Autodesk Fusion 360 part; units mm, degrees
sketch "Sketch1" plane through (0, 0, 0) normal (0, 0, 1) x (1, 0, 0)
  line L0 (12.75, -12.75) -> (-12.75, -12.75)
  line L1 (-12.75, -12.75) -> (-12.75, 12.75)
  line L2 (-12.75, 12.75) -> (12.75, 12.75)
  line L3 (12.75, 12.75) -> (12.75, -12.75)
  line L4 (12.75, -12.75) -> (-12.75, 12.75) construction
  line L5 (-12.75, -12.75) -> (12.75, 12.75) construction
  line L6 (-0.75, 12.75) -> (0.75, 12.75)
  line L7 (0.75, 12.75) -> (0.75, 42.75)
  line L8 (0.75, 42.75) -> (-0.75, 42.75)
  line L9 (-0.75, 42.75) -> (-0.75, 12.75)
  dimension "d1" = 25.5
  dimension "d2" = 25.5
  dimension "d3" = 1.5
  dimension "d4" = 30
  dimension "d5" = 0.75
extrude "Extrude1" add sketch "Sketch1" along normal blind 10 makes body 1
sketch "Sketch2" plane through (0, 0, 10) normal (0, 0, 1) x (-1, 0, 0)
  line L0 (-0.75, -12.75) -> (-0.75, -42.75)
  line L1 (-0.75, -42.75) -> (0.75, -42.75)
  line L2 (0.75, -42.75) -> (0.75, -12.75)
  line L3 (0.75, -12.75) -> (12.75, -12.75)
  line L4 (12.75, -12.75) -> (12.75, 12.75)
  line L5 (12.75, 12.75) -> (-12.75, 12.75)
  line L6 (-12.75, 12.75) -> (-12.75, -12.75)
  line L7 (-12.75, -12.75) -> (-0.75, -12.75)
  line L8 (-15, 15) -> (15, 15)
  line L9 (15, 15) -> (15, -15)
  line L10 (15, -15) -> (-15, -15)
  line L11 (-15, -15) -> (-15, 15)
  line L12 (-15, 15) -> (15, -15) construction
  line L13 (15, 15) -> (-15, -15) construction
  line L14 (-22.5, 15) -> (22.5, 15)
  line L15 (22.5, 15) -> (22.5, -15)
  line L16 (22.5, -15) -> (-22.5, -15)
  line L17 (-22.5, -15) -> (-22.5, 15)
  line L18 (-22.5, 15) -> (22.5, -15) construction
  line L19 (22.5, 15) -> (-22.5, -15) construction
  line L20 (-26.5, 6.65) -> (-18.5, 6.65)
  line L21 (-18.5, 6.65) -> (-18.5, -6.65)
  line L22 (-18.5, -6.65) -> (-26.5, -6.65)
  line L23 (-26.5, -6.65) -> (-26.5, 6.65)
  line L24 (-26.5, 6.65) -> (-18.5, -6.65) construction
  line L25 (-18.5, 6.65) -> (-26.5, -6.65) construction
  line L26 (18.5, 6.65) -> (26.5, 6.65)
  line L27 (26.5, 6.65) -> (26.5, -6.65)
  line L28 (26.5, -6.65) -> (18.5, -6.65)
  line L29 (18.5, -6.65) -> (18.5, 6.65)
  line L30 (18.5, 6.65) -> (26.5, -6.65) construction
  line L31 (26.5, 6.65) -> (18.5, -6.65) construction
  point P0 (-22.5, 0)
  point P1 (22.5, 0)
  dimension "d8" = 30
  dimension "d9" = 30
  dimension "d10" = 45
  dimension "d11" = 30
  dimension "d12" = 8
  dimension "d13" = 13.3
  dimension "d14" = 8
  dimension "d15" = 13.3
extrude "Extrude2" add sketch "Sketch2" against normal blind 10 separate body contours L0 L2 L3 L4 L5 L6 L7 L8 L9 L10 L11 L14 L16 makes body 2
extrude "Extrude3" add sketch "Sketch2" along normal blind 1.5 contours L0 L2 L3 L4 L5 L6 L7 L10 L16 | L0 L2 L3 L4 L5 L6 L7 L8 L9 L10 L11 L14 L16 | L11 L14 L16 L17 L20 L21 L22 | L9 L14 L15 L16 L26 L28 L29 | L17 L20 L21 L22 | L15 L26 L28 L29 bodies 2
extrude "Extrude4" add sketch "Sketch2" against normal blind 0.7 contours L11 L14 L16 L17 L20 L21 L22 | L9 L14 L15 L16 L26 L28 L29 bodies 2
extrude "Extrude5" add sketch "Sketch2" against normal blind 1.5 from surface at -0.7 contours L11 L14 L16 L17 L20 L21 L22 | L9 L14 L15 L16 L26 L28 L29 | L17 L20 L21 L22 | L15 L26 L28 L29 bodies 2
hidden bodies 1
The model under review builds one solid part; all positions refer to its coordinate system, in mm. A direction names the side the tool comes from. Round coordinates to 2 decimals unless told otherwise and drop trailing zeros. Write each loop counter-clockwise with the first axis right and the second up, starting at its lowest first coordinate (ties: lowest second). Pieces come first, ordered by that corner, then holes.
(1) Insertion check: pin 1 (1.5 mm diameter, centred on x = -2, y = 10, fed in from -Z); pin 2 (1.2 mm diameter, centred on x = -21.5, y = -3, fed in from -Z). Each pin has a flat end and moves straight along its axis. Give the tip position at first contact, or say it passes through.
(2) We need section B-B on z = 7.25. Give the boundary of the cut face in (x, y), and give its area (3 significant figures).
(3) We need section A-A on x = 19. Give the boundary of the cut face in (y, z), and give its area (3 significant figures).
(4) Mouldability with a two-part tool opening along Y and no side actions: class faces 1 (the flat face through (0, -12.75, 5)), 2 (the flat face through (-12.75, 0, 5)), 3 (the flat face through (5, 15, 7)), 4 (the flat face through (-19, 0, 7.8)) as +Y half, -Y half, draft (parallel to the pull), parting line (faces both ways), or undercut.
(5) We need section C-C on y = -5. Give the boundary of the cut face in (x, z).
(6) Machinability: for faces 5 (the flat face through (19, 0, 7.8)), 6 (the flat face through (7, 12.75, 5)), 7 (the flat face through (21, 0, 10)), which of the approach directions +Z, -Z, +X, -X, +Y, -Y give a long, thin tool a straight path to every point of the face, cutting with its end or side? Answer none if there is none.
(7) We need section D-D on x = 5.5. Give the boundary of the cut face in (y, z).
(8) Wall thickness on L1, parallel to X at y = -11, z = 2.5; L2, parallel to X at y = 8.75, z = 9.5: over which ranges is each line inside the solid? List them lowest first.
Findings below:
1. pin 1: stops at z = 10
1. pin 2: stops at z = 7.8
2. outline: (-15, -15) - (15, -15) - (15, 15) - (0.75, 15) - (0.75, 12.75) - (12.75, 12.75) - (12.75, -12.75) - (-12.75, -12.75) - (-12.75, 12.75) - (-0.75, 12.75) - (-0.75, 15) - (-15, 15) - close
2. area: 246 mm2
3. outline: (-15, 7.8) - (15, 7.8) - (15, 11.5) - (-15, 11.5) - close; hole (-6.65, 9.3) - (6.65, 9.3) - (6.65, 10) - (-6.65, 10) - close
3. area: 102 mm2
4. face 1: undercut
4. face 2: undercut
4. face 3: +Y half
4. face 4: draft
5. outline: (-22.5, 7.8) - (-15, 7.8) - (-15, 0) - (-12.75, 0) - (-12.75, 10) - (12.75, 10) - (12.75, 0) - (15, 0) - (15, 7.8) - (22.5, 7.8) - (22.5, 9.3) - (18.5, 9.3) - (18.5, 10) - (22.5, 10) - (22.5, 11.5) - (-22.5, 11.5) - (-22.5, 10) - (-18.5, 10) - (-18.5, 9.3) - (-22.5, 9.3) - close
6. face 5: -Z, +X, +Y, -Y
6. face 6: -Z
6. face 7: +X
7. outline: (-15, 0) - (-12.75, 0) - (-12.75, 10) - (12.75, 10) - (12.75, 0) - (15, 0) - (15, 11.5) - (-15, 11.5) - close
8. L1: x = -15 to -12.75, 12.75 to 15
8. L2: x = -22.5 to -12.75, 12.75 to 22.5
